Work out the finished part from the listing and answer in its coordinate system (mm). A direction names the side the tool comes from. Round coordinates to 2 decimals unless told otherwise and drop trailing zeros. Write each loop counter-clockwise with the first axis right and the second up, starting at its lowest first coordinate (ties: lowest second). Pieces come first, ordered by that corner, then holes. Notation, with made-up numbers: (30.5, 45.25) - (73.5, 45.25) arc R33 cw to (73.5, 83.25) - close; hole circle Ø4 at (41, 85.25). An arc over 180 degrees is marked (long way). Answer as a JSON object with one key per item and string values.
```python
from build123d import *

# Parameters (mm, degrees)
SKETCH_1_W          = 65
SKETCH_1_H          = 120
EXTRUDE_1_DEPTH     = 3
SKETCH_2_W          = 2
SKETCH_2_H          = 120
EXTRUDE_2_DEPTH     = 8.75
FILLET_1_R          = 2
SKETCH_3_R          = 1.5
CUT_EXTRUDE_1_DEPTH = 70.240974141
SKETCH_4_R          = 1.5
CUT_EXTRUDE_2_DEPTH = 90.235993299


with BuildPart() as part:
    # 草图1 → 凸台-拉伸1 (new body)
    with BuildSketch(Plane(origin=(0, 0, 0), x_dir=(1, 0, 0), z_dir=(0, 1, 0))):
        Rectangle(SKETCH_1_W, SKETCH_1_H)
    extrude(amount=EXTRUDE_1_DEPTH)

    # 草图2 → 凸台-拉伸2 (add)
    with BuildSketch(Plane(origin=(0, 3, 0), x_dir=(1, 0, 0), z_dir=(0, 1, 0))):
        with Locations((-31.5, 0)):
            Rectangle(SKETCH_2_W, SKETCH_2_H)
        with Locations((31.5, 0)):
            Rectangle(SKETCH_2_W, SKETCH_2_H)
    extrude(amount=EXTRUDE_2_DEPTH)

    # 圆角1
    fillet_1_edges = [part.edges().sort_by_distance(p)[0] for p in [
        (-32.5, 0, 0),
        (32.5, 0, 0),
    ]]
    fillet(fillet_1_edges, radius=FILLET_1_R)

    # 草图3 → 切除-拉伸1 (cut, through all)
    with BuildSketch(Plane.XZ):
        with Locations(Location((-15, 40, 0), (0, 0, 270))):
            Circle(SKETCH_3_R)
        with Locations(Location((15, 40, 0), (0, 0, 270))):
            Circle(SKETCH_3_R)
        with Locations(Location((-15, 20, 0), (0, 0, 270))):
            Circle(SKETCH_3_R)
        with Locations(Location((15, 20, 0), (0, 0, 270))):
            Circle(SKETCH_3_R)
        with Locations(Location((-15, 0, 0), (0, 0, 270))):
            Circle(SKETCH_3_R)
        with Locations(Location((15, 0, 0), (0, 0, 270))):
            Circle(SKETCH_3_R)
        with Locations(Location((-15, -20, 0), (0, 0, 270))):
            Circle(SKETCH_3_R)
        with Locations(Location((15, -20, 0), (0, 0, 270))):
            Circle(SKETCH_3_R)
        with Locations(Location((-15, -40, 0), (0, 0, 270))):
            Circle(SKETCH_3_R)
        with Locations(Location((15, -40, 0), (0, 0, 270))):
            Circle(SKETCH_3_R)
    extrude(amount=-CUT_EXTRUDE_1_DEPTH, mode=Mode.SUBTRACT)

    # 草图4 → 切除-拉伸2 (cut, through all)
    with BuildSketch(Plane.ZY.offset(32.5)):
        with Locations((0, 6.75)):
            Circle(SKETCH_4_R)
        with Locations((-20, 6.75)):
            Circle(SKETCH_4_R)
        with Locations((-40, 6.75)):
            Circle(SKETCH_4_R)
        with Locations((20, 6.75)):
            Circle(SKETCH_4_R)
        with Locations((40, 6.75)):
            Circle(SKETCH_4_R)
    extrude(amount=-CUT_EXTRUDE_2_DEPTH, mode=Mode.SUBTRACT)


solid = part.part
```
Item 1: A cutting plane is placed at B-B (z = 40). Write down the section's boundary in (x, y).
Results found:
{"outline": "(-32.5, 2) arc R2 ccw to (-30.5, 0) - (-16.5, 0) - (-16.5, 3) - (-30.5, 3) - (-30.5, 5.25) - (-32.5, 5.25) - close; (-32.5, 8.25) - (-30.5, 8.25) - (-30.5, 11.75) - (-32.5, 11.75) - close; (-13.5, 0) - (13.5, 0) - (13.5, 3) - (-13.5, 3) - close; (16.5, 0) - (30.5, 0) arc R2 ccw to (32.5, 2) - (32.5, 5.25) - (30.5, 5.25) - (30.5, 3) - (16.5, 3) - close; (30.5, 8.25) - (32.5, 8.25) - (32.5, 11.75) - (30.5, 11.75) - close"}
Item 2: A cutting plane is placed at A-A (x = -15). Write down the section's boundary in (y, z), and give its area (3 significant figures).
Results found:
{"outline": "(0, -60) - (3, -60) - (3, -41.5) - (0, -41.5) - close; (0, -38.5) - (3, -38.5) - (3, -21.5) - (0, -21.5) - close; (0, -18.5) - (3, -18.5) - (3, -1.5) - (0, -1.5) - close; (0, 1.5) - (3, 1.5) - (3, 18.5) - (0, 18.5) - close; (0, 21.5) - (3, 21.5) - (3, 38.5) - (0, 38.5) - close; (0, 41.5) - (3, 41.5) - (3, 60) - (0, 60) - close", "area": "315 mm²"}
Item 3: Determine the mould class of faces 1 (the cylindrical face through (-14.93, 1.48, 41.5)), 2 (the cylindrical face through (31.49, 5.84, 38.81)), 3 (the flat face through (32.5, 9, 1)) for opening direction X: pulls with the +X half, pulls with the -X half, needs draft (parallel to the pull), parting line crosses it, or undercut.
Results found:
{"face 1": "undercut", "face 2": "needs draft", "face 3": "pulls with the +X half"}
Item 4: A cutting plane is placed at C-C (z = 3.5). Write down the section's boundary in (x, y).
Results found:
{"outline": "(-32.5, 2) arc R2 ccw to (-30.5, 0) - (30.5, 0) arc R2 ccw to (32.5, 2) - (32.5, 11.75) - (30.5, 11.75) - (30.5, 3) - (-30.5, 3) - (-30.5, 11.75) - (-32.5, 11.75) - close"}
Item 5: A cutting plane is placed at D-D (y = 6.75). Give the number of separate pieces and of enclosed holes in the cut face, and give its area (3 significant figures).
Results found:
{"separate pieces": "12", "enclosed holes": "0", "area": "420 mm²"}
Item 6: This flat-tipped pin is pushed along its axis until it touches: P1, Ø8, axis at x = -19, z = 11.5, coming from the +Y side. Where does it stop, or does it pass through?
Results found:
{"P1": "y = 3"}
Item 7: Consider line 1 along X through (y, z) = (2.3, -40); line 2 along X through (y, z) = (1.4, 20); line 3 along X through (y, z) = (3.5, -17). Determine where each line is inside the solid, lowest interval first.
Results found:
{"line 1": "-32.5 to -16.5, -13.5 to 13.5, 16.5 to 32.5", "line 2": "-32.41 to -16.5, -13.5 to 13.5, 16.5 to 32.41", "line 3": "-32.5 to -30.5, 30.5 to 32.5"}
Item 8: For faces 4 (the cylindrical face through (15.07, 1.48, 41.5)), 5 (the flat face through (30.5, 8.3, 0.8)), determine the directions among +Z, -Z, +X, -X, +Y, -Y from which every point of the face is accessible in a straight line to the end or side of a thin tool.
Results found:
{"face 4": "+Y, -Y", "face 5": "+Z, -Z, +Y"}
